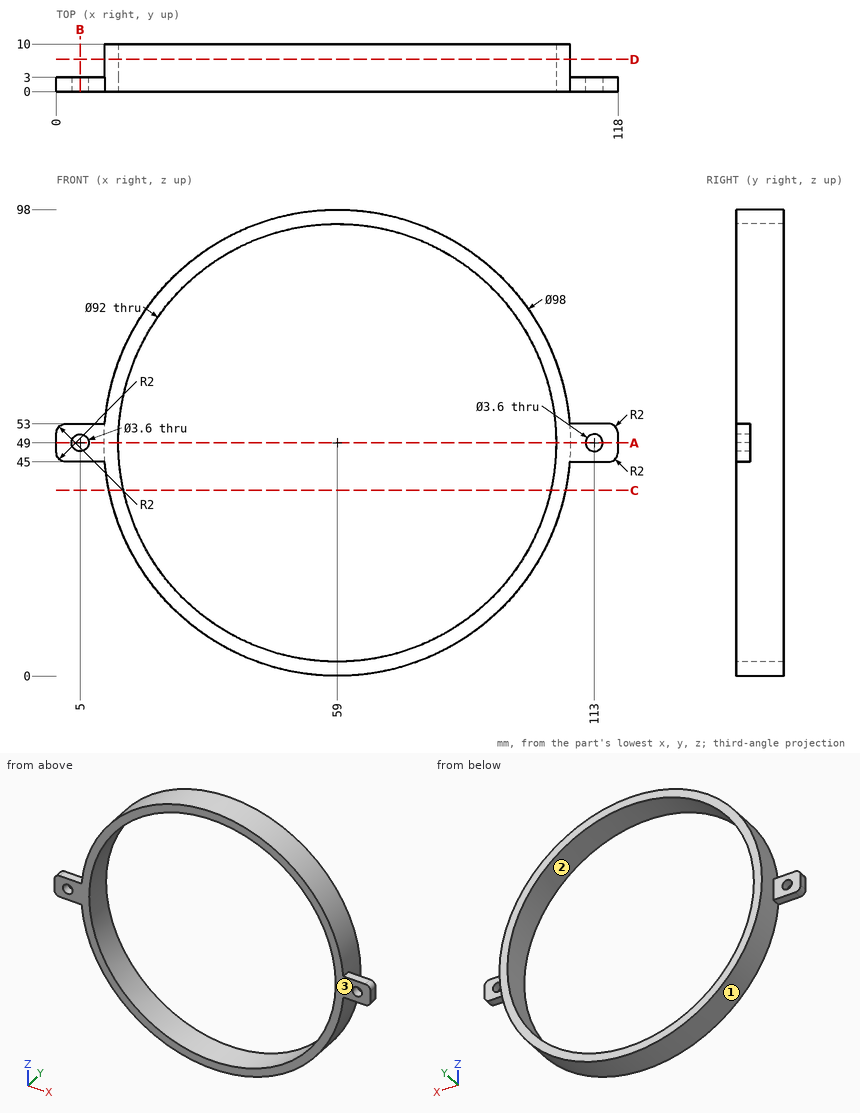
Input: dimensioned drawing with shaded views. Units: mm. Origin: part minimum x, y, z. Coordinates: 2 decimals unless noted, no trailing zeros. Loops run counter-clockwise (first coordinate to the right, second up) from the corner with the lowest first, then second, coordinate; pieces in that order, holes last. Notation, with made-up numbers: M -32,-20 L 14,-20 A16 cw 14,5 Z; hole C 31.25,-33 d9. An arc over 180 degrees is marked long. Use a Markdown table: item, result. Add a question column.
1) Pin query (flat end, axial travel): P1, Ø3, axis at x = 84, y = 5.5, coming from the +Z side; P2, Ø1.5, axis at x = 5, y = 1, coming from the +Z side; P3, Ø1.5, axis at y = 3, z = 19.5, coming from the +X side; P4, Ø6, axis at x = 113, z = 49, coming from the -Y side. Return the tip coordinate at first contact, or that it passes through.
2) Section A-A, the plane z = 49. Return the cut outline in (x, y).
3) Section D-D, the plane y = 6.75. Return the cut outline in (x, z).
4) Section B-B, the plane x = 5. Return the cut outline in (y, z), plus the area to 3 significant figures.
5) Draft query along Z for the marked faces 1, 2 and 3. Return one class per face: +Z half, -Z half, draft (parallel to the pull), parting line (faces both ways), or undercut.
6) Section C-C, the plane z = 39. Return the cut outline in (x, y), plus the area to 3 significant figures.
7) Line query: L1, parallel to X at y = 1.3, z = 49; L2, parallel to Z at x = 113, y = 2.35; L3, parallel to X at y = 8, z = 49. Output: solid intervals per line, ascending. Write a range as from..to.
Answer below:
| question | item | result |
|---|---|---|
| 1 | P1 | z = 92 |
| 1 | P2 | z = 53 |
| 1 | P3 | x = 98.68 |
| 1 | P4 | y = 0 |
| 2 | outline | M 0,0 L 3.2,0 L 3.2,3 L 0,3 Z; M 6.8,0 L 13,0 L 13,10 L 10,10 L 10,3 L 6.8,3 Z; M 105,0 L 111.2,0 L 111.2,3 L 108,3 L 108,10 L 105,10 Z; M 114.8,0 L 118,0 L 118,3 L 114.8,3 Z |
| 3 | outline | C 59,49 d98; hole C 59,49 d92 |
| 4 | outline | M 0,45 L 3,45 L 3,47.2 L 0,47.2 Z; M 0,50.8 L 3,50.8 L 3,53 L 0,53 Z |
| 4 | area | 13.2 mm2 |
| 5 | face 1 | parting line |
| 5 | face 2 | undercut |
| 5 | face 3 | draft |
| 6 | outline | M 11.03,0 L 14.1,0 L 14.1,10 L 11.03,10 Z; M 103.9,0 L 106.97,0 L 106.97,10 L 103.9,10 Z |
| 6 | area | 61.4 mm2 |
| 7 | L1 | 0..3.2, 6.8..13, 105..111.2, 114.8..118 |
| 7 | L2 | 45..47.2, 50.8..53 |
| 7 | L3 | 10..13, 105..108 |
